Can you work these out from the model? Positions are in its coordinate system, mm. A direction names the side the tool comes from. Coordinates: 2 decimals unless noted, no trailing zeros. Order: outer loops, then holes, each group sorted by start corner. A loop starts at its lowest first (then second) coordinate and runs counter-clockwise, first axis right, second up. Notation, with made-up numbers: (82.25, 17.25) -> (104.25, 17.25) arc R9 ccw to (104.25, 24.25) -> close; hole circle Ø7 at (3.25, 42.25). An arc over 180 degrees is marked (long way). Answer as a JSON object with one key per item and string values. Group by question number.
(1) Which directions (+Z, -Z, +X, -X, +Y, -Y) give clear straight access to the entire face, cutting with the end or side of a thin tool? Please do faces 1 (the flat face through (-29.12, -0.07, 19.08)), 2 (the flat face through (-19, -4.762, 31)).
(2) If we mould it in two halves opening along X, with no side actions, what happens to faces 3 (the flat face through (-25, 0, 0)), 4 (the flat face through (-18.068, 0, 25)), 5 (the flat face through (-50.8, 0, 25))? For each: pulls with the +X half, pulls with the -X half, needs draft (parallel to the pull), parting line crosses it, or undercut.
(3) I need wall thicknesses on line 1 (X direction, y = -0.5, z = 23.5); line 2 (X direction, y = 2.5, z = 32); line 3 (Z direction, x = -31, y = -4.25). Which ranges of each line are inside material? Lowest first, please.
(4) I want a section at B-B, the plane z = 27.5. List the corners of the cut face in (x, y) for me.
(5) I want a section at A-A, the plane y = -0.25. List the corners of the cut face in (x, z) for me.
Autodesk Inventor part; units mm, degrees
ref_plane "YZ Plane" through (0, 0, 0) normal (1, 0, 0) x (0, 1, 0)
ref_plane "XZ Plane" through (0, 0, 0) normal (0, 1, 0) x (-1, 0, 0)
ref_plane "XY Plane" through (0, 0, 0) normal (0, 0, 1) x (1, 0, 0)
sketch "Sketch1" plane through (0, 0, 0) normal (0, 1, 0) x (-1, 0, 0)
  line L0 (50.8, 0) -> (50.8, 50.8)
  line L1 (50.8, 50.8) -> (0, 50.8)
  line L2 (0, 50.8) -> (0, 0)
  line L3 (0, 0) -> (50.8, 0)
  line L4 (25.4, 16.9333) -> (18.0677, 21.1667)
  line L5 (18.0677, 21.1667) -> (18.0677, 29.6333)
  line L6 (18.0677, 29.6333) -> (25.4, 33.8667)
  line L7 (25.4, 33.8667) -> (32.7323, 29.6333)
  line L8 (32.7323, 29.6333) -> (32.7323, 21.1667)
  line L9 (32.7323, 21.1667) -> (25.4, 16.9333)
  point P0 (25.4, 25.4)
  point P1 (21.7338, 19.05)
  point P2 (29.0662, 31.75)
  dimension "d0" = 50.8
  dimension "d1" = 50.8
  dimension "d4" = 12.7
extrude "Extrusion1" add sketch "Sketch1" along normal mid plane 9.525
properties part number "Hex Box"
Computed values:
{
 "1": {"face 1": "+Y, -Y", "face 2": "+Z, -Z, +X, -X, -Y"},
 "2": {"face 3": "needs draft", "face 4": "undercut", "face 5": "pulls with the -X half"},
 "3": {"line 1": "x = -50.8 to -32.73, -18.07 to 0", "line 2": "x = -50.8 to -28.63, -22.17 to 0", "line 3": "z = 0 to 20.17, 30.63 to 50.8"},
 "4": {"outline": "(-50.8, -4.76) -> (-32.73, -4.76) -> (-32.73, 4.76) -> (-50.8, 4.76) -> close; (-18.07, -4.76) -> (0, -4.76) -> (0, 4.76) -> (-18.07, 4.76) -> close"},
 "5": {"outline": "(-50.8, 0) -> (0, 0) -> (0, 50.8) -> (-50.8, 50.8) -> close; hole (-32.73, 21.17) -> (-25.4, 16.93) -> (-18.07, 21.17) -> (-18.07, 29.63) -> (-25.4, 33.87) -> (-32.73, 29.63) -> close"}
}
